Geometry check sheet. Reference: drawing and pictorial views, mm from the part's lowest x, y, z. Give positions to 0.01 mm unless a question says otherwise; leave off trailing zeros. Write each loop counter-clockwise with the first axis right and the second up, starting at its lowest first coordinate (ties: lowest second). Pieces come first, ordered by that corner, then holes. Notation, with made-up numbers: M 8,-18.75 L 17,-18.75 A24 ccw 17,9.25 Z; hole C -24.5,6.25 d3. An arc over 180 degrees is marked long. One line per item, written item: value. Start each with the question number.
1. Scan lines: line 1 (X direction, y = 3.75, z = 55); line 2 (Y direction, x = 3, z = 19). Record each from-to range of solid material in increasing order.
2. Gauge pin test, flat ends, axial feed: pin 1 (1.4 mm diameter, centred on y = 3, z = 12.5, fed in from -X); pin 2 (2.5 mm diameter, centred on x = 31, y = 4.5, fed in from -Z); pin 3 (3 mm diameter, centred on x = 42, z = 27, fed in from -Y); pin 4 (2.5 mm diameter, centred on y = 3.5, z = 27, fed in from +X). Record the tip position at first contact, or that the pin passes through.
3. Cross-section at B-B on x = 24.5. Record the cut outline in (y, z), then the cut area to 3 significant figures.
4. Cross-section at C-C on y = 5.25. Count the separate pieces of the cut face and the enclosed holes in it, then the cut area to 4 significant figures.
5. Cross-section at A-A on z = 25.5. Record the cut outline in (x, y).
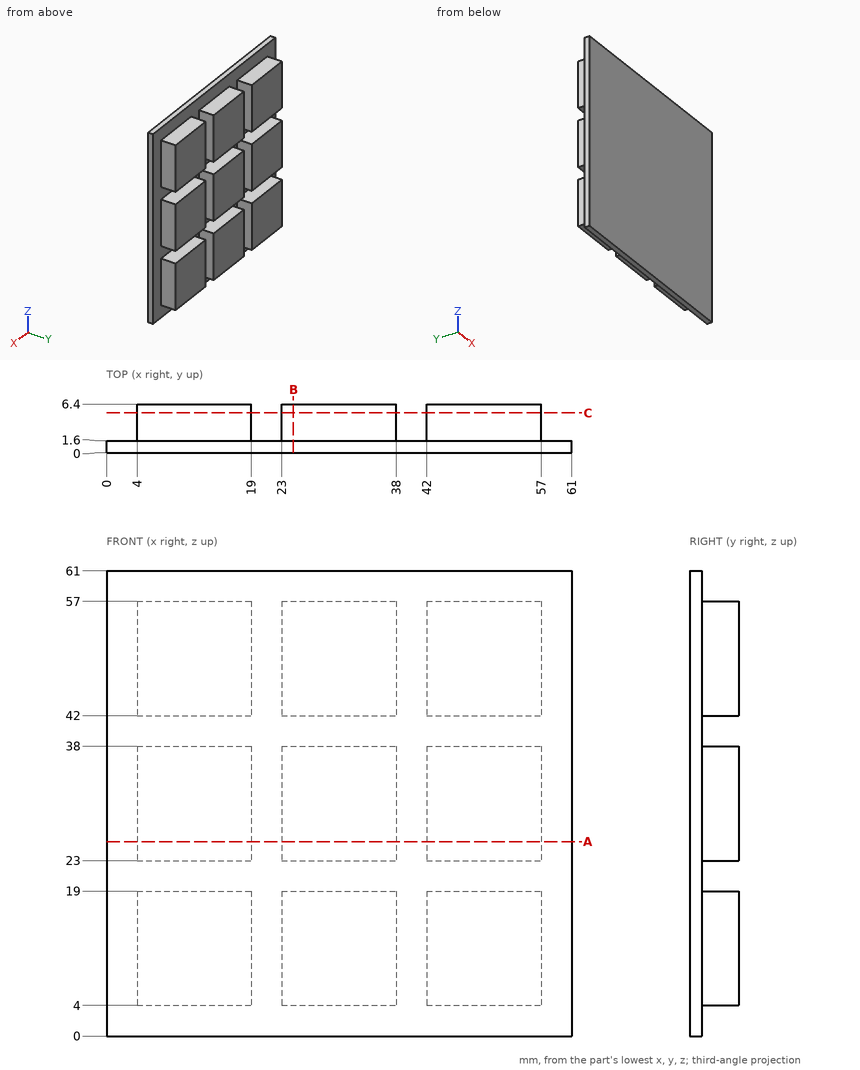
Report:
1. line 1: x = 4 to 19, 23 to 38, 42 to 57
1. line 2: y = 0 to 1.6
2. pin 1: stops at x = 4
2. pin 2: stops at z = 4
2. pin 3: stops at y = 0
2. pin 4: stops at x = 57
3. outline: M 0,0 L 1.6,0 L 1.6,4 L 6.4,4 L 6.4,19 L 1.6,19 L 1.6,23 L 6.4,23 L 6.4,38 L 1.6,38 L 1.6,42 L 6.4,42 L 6.4,57 L 1.6,57 L 1.6,61 L 0,61 Z
3. area: 314 mm^2
4. separate pieces: 9
4. enclosed holes: 0
4. area: 2,025 mm^2
5. outline: M 0,0 L 61,0 L 61,1.6 L 57,1.6 L 57,6.4 L 42,6.4 L 42,1.6 L 38,1.6 L 38,6.4 L 23,6.4 L 23,1.6 L 19,1.6 L 19,6.4 L 4,6.4 L 4,1.6 L 0,1.6 Z
